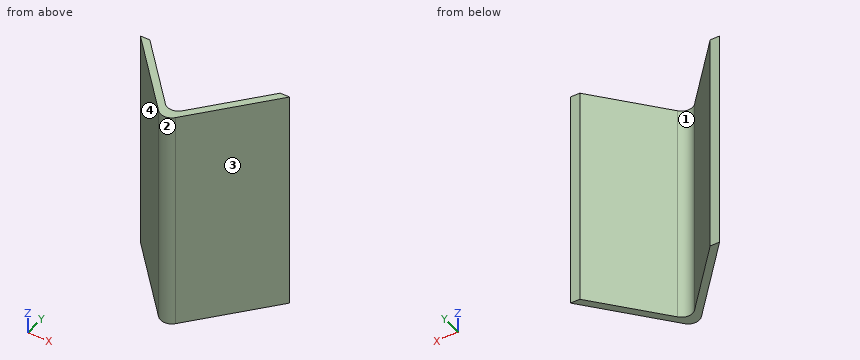
```python
from build123d import *

# Parameters (mm, degrees)
F1_DEPTH = 101.6
F2_R     = 5.08
F3_R     = 5.08


with BuildPart() as f1:
    # F0 (on Top) → F1 (new body)
    with BuildSketch(Plane.XY):
        Polygon((-33.663134, 0), (0, -38.04515), (33.663134, 0), (29.423697, 0), (0, -33.253855), (-29.423697, 0), align=None)
    extrude(amount=F1_DEPTH)

    # F2
    f2_edges = [f1.edges().sort_by_distance(p)[0] for p in [
        (0, -33.253855, 50.8),
    ]]
    fillet(f2_edges, radius=F2_R)

    # F3
    f3_edges = [f1.edges().sort_by_distance(p)[0] for p in [
        (0, -38.04515, 50.8),
    ]]
    fillet(f3_edges, radius=F3_R)


solid = f1.part
```
CAD build for the part. Positions are in the model's coordinates, mm. Face numbers are marked on the shaded views. Round coordinates to 2 decimals unless told otherwise and drop trailing zeros. Loops run counter-clockwise (first coordinate to the right, second up) from the corner with the lowest first, then second, coordinate; pieces in that order, holes last. Notation, with made-up numbers: (23, -0.75) - (44, -0.75) arc R15 ccw to (44, 25.25) - close; hole circle Ø2 at (21, 50.5). An arc over 180 degrees is marked (long way). Return JSON: item names as keys, results as strings. Group by question number.
Q1. Band-saw the part on B-B on y = -5.5. Give the cut face in (x, z).
Q2. Flat gauge pins, fed straight in: pin 1 Ø3 at (x, y) = (-1, -28) entering from +Z; pin 2 Ø3 at (x, z) = (-9.5, 84) entering from +Y; pin 3 Ø6 at (x, z) = (12, 78) entering from -Y; pin 4 Ø6 at (x, z) = (-7.5, 31.5) entering from -Y. Where does each tip first touch, or does it go through?
Q3. Two-plate mould, pull along X, no slides. Class the marked faces 1, 2, 3 and 4: +X half, -X half, draft (parallel to the pull), parting line (faces both ways), or undercut.
Q4. Drill centre lines: line 1 along X through (y, z) = (-16, 27); line 2 along X through (y, z) = (-26.5, 13); line 3 along Y through (x, z) = (-3.5, 39). Where is each one in solid material? Low to high. Write a range as [from, to].
Q5. Band-saw the part on C-C on x = -0.5. Give the cut face in (y, z), plus the area to 3 significant figures.
Q6. Band-saw the part on A-A on z = 23.5. Give the cut face in (x, y), plus the area to 3 significant figures.
Solutions:
{
 "1": {"outline": "(-28.8, 0) - (-24.56, 0) - (-24.56, 101.6) - (-28.8, 101.6) - close; (24.56, 0) - (28.8, 0) - (28.8, 101.6) - (24.56, 101.6) - close"},
 "2": {"pin 1": "passes through", "pin 2": "stops at y = -20.82", "pin 3": "stops at y = -27.87", "pin 4": "stops at y = -32.96"},
 "3": {"face 1": "undercut", "face 2": "parting line", "face 3": "+X half", "face 4": "-X half"},
 "4": {"line 1": "x = [-19.51, -15.27], [15.27, 19.51]", "line 2": "x = [-10.22, -5.98], [5.98, 10.22]", "line 3": "y = [-34.06, -29.27]"},
 "5": {"outline": "(-35.43, 0) - (-30.64, 0) - (-30.64, 101.6) - (-35.43, 101.6) - close", "area": "487 mm^2"},
 "6": {"outline": "(-33.66, 0) - (-3.8, -33.75) arc R5.08 ccw to (3.8, -33.75) - (33.66, 0) - (29.42, 0) - (3.8, -28.95) arc R5.08 cw to (-3.8, -28.95) - (-29.42, 0) - close", "area": "302 mm^2"}
}
